Geometry check sheet. Reference: drawing and pictorial views, mm from the part's lowest x, y, z. Give positions to 0.01 mm unless a question says otherwise; leave off trailing zeros. Order: outer loops, then holes, each group sorted by start corner. A loop starts at its lowest first (then second) coordinate and runs counter-clockwise, first axis right, second up.
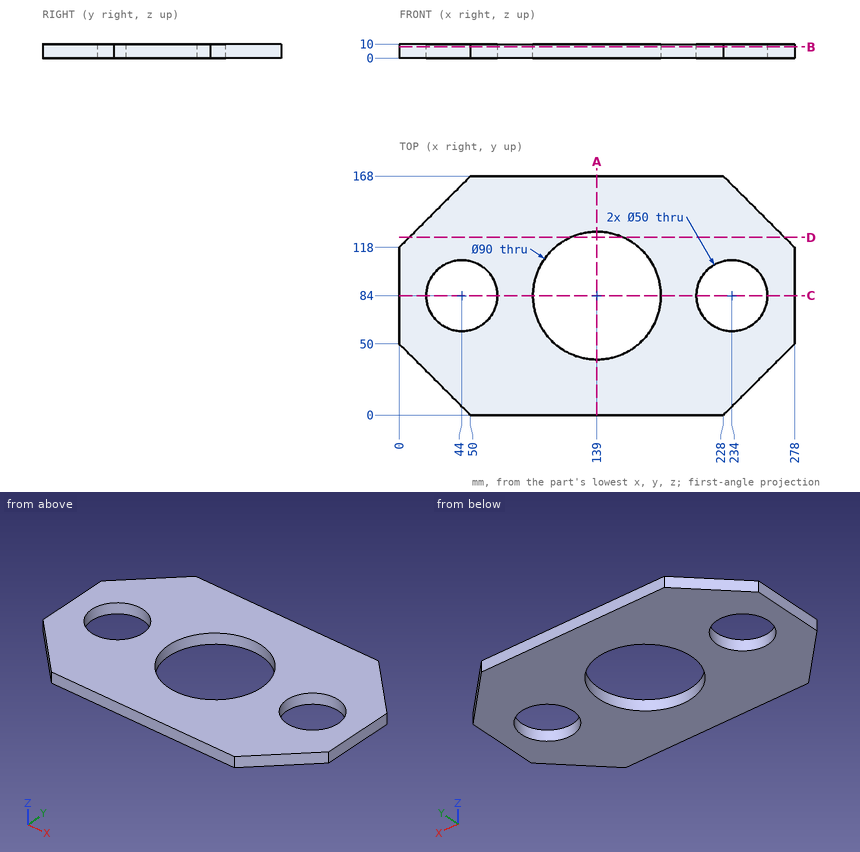
1) Material ranges on L1, parallel to X at y = 84, z = 5.25; L2, parallel to Y at x = 139, z = 1.25; L3, parallel to Y at x = 170, z = 8, recorded low to high.
Recorded:
L1: x = 0 to 19, 69 to 94, 184 to 209, 259 to 278
L2: y = 0 to 39, 129 to 168
L3: y = 0 to 51.38, 116.62 to 168
2) Depth check by flat-ended pin: pin 1 Ø4 at (x, y) = (87, 68) entering from -Z; pin 2 Ø1 at (y, z) = (123.5, 4) entering from +X; pin 3 Ø3 at (y, z) = (33.5, 7.5) entering from -X. Enter the tip coordinate at first touch or a pass-through.
Recorded:
pin 1: stops at z = 0
pin 2: stops at x = 273
pin 3: stops at x = 15
3) Section check D-D, the plane y = 125. Record the cut outline in (x, z), then the cut area to 3 significant figures.
Recorded:
outline: (7, 0) - (120.45, 0) - (120.45, 10) - (7, 10) - close; (157.55, 0) - (271, 0) - (271, 10) - (157.55, 10) - close
area: 2,270 mm2
4) Section check C-C, the plane y = 84. Record the cut outline in (x, z), then the cut area to 3 significant figures.
Recorded:
outline: (0, 0) - (19, 0) - (19, 10) - (0, 10) - close; (69, 0) - (94, 0) - (94, 10) - (69, 10) - close; (184, 0) - (209, 0) - (209, 10) - (184, 10) - close; (259, 0) - (278, 0) - (278, 10) - (259, 10) - close
area: 880 mm2
5) Section check B-B, the plane z = 8. Record the cut outline in (x, y), then the cut area to 3 significant figures.
Recorded:
outline: (0, 50) - (50, 0) - (228, 0) - (278, 50) - (278, 118) - (228, 168) - (50, 168) - (0, 118) - close; hole circle Ø50 at (44, 84); hole circle Ø90 at (139, 84); hole circle Ø50 at (234, 84)
area: 31,400 mm2
6) Section check A-A, the plane x = 139. Record the cut outline in (y, z), then the cut area to 3 significant figures.
Recorded:
outline: (0, 0) - (39, 0) - (39, 10) - (0, 10) - close; (129, 0) - (168, 0) - (168, 10) - (129, 10) - close
area: 780 mm2
